Could you check a few things on this drawing? It's one solid part, dimensions in mm from its lowest x, y, z. A direction names the side the tool comes from. Give positions to 0.01 mm unless a question says otherwise; leave off trailing zeros. Order: outer loops, then holes, each group sorted by start corner. A loop starts at its lowest first (then second) coordinate and runs counter-clockwise, first axis right, second up.
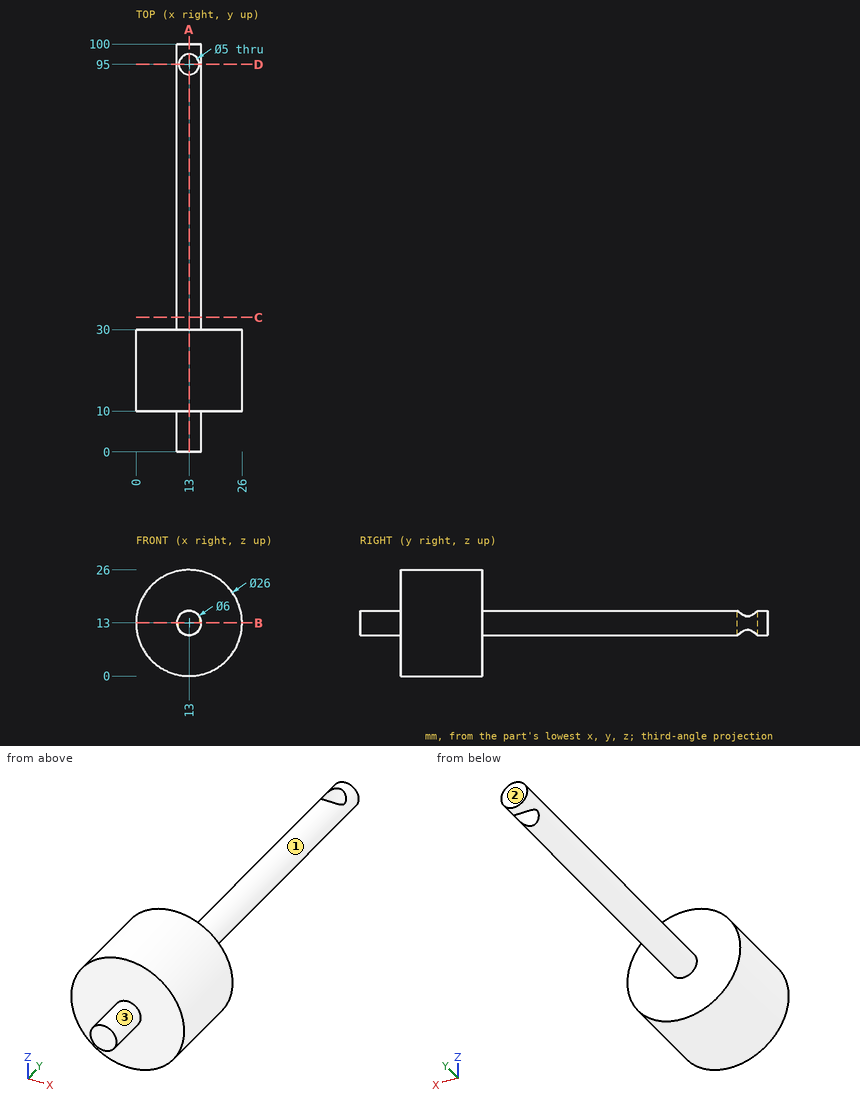
Q1. If we section it at B-B on z = 13: List the corners of the cut face in (x, y) for me.
Filled sheet:
outline: (0, 10) - (10, 10) - (10, 0) - (16, 0) - (16, 10) - (26, 10) - (26, 30) - (16, 30) - (16, 100) - (10, 100) - (10, 30) - (0, 30) - close; hole circle Ø5 at (13, 95)
Q2. I need wall thicknesses on L1, parallel to Y at x = 9.5, z = 6.75; L2, parallel to X at y = 95, z = 13.25; L3, parallel to Y at x = 13, z = 14. Which ranges of each line are inside material? Lowest first, please.
Filled sheet:
L1: y = 10 to 30
L2: x = 10.01 to 10.5, 15.5 to 15.99
L3: y = 0 to 92.5, 97.5 to 100
Q3. I'm going to push flat-ended pins straight in: P1, Ø12, axis at x = 19, y = 74, coming from the +Z side; P2, Ø8, axis at x = 6.5, y = 58, coming from the -Z side; P3, Ø12, axis at x = 5, z = 12.5, coming from the +Y side; P4, Ø5, axis at x = 20, z = 9, coming from the +Y side. Where does each tip first touch, or does it pass through?
Filled sheet:
P1: stops at z = 16
P2: stops at z = 11.34
P3: stops at y = 100
P4: stops at y = 30
Q4. If we section it at C-C on y = 33: List the corners of the cut face in (x, z) for me, plus the area to 3 significant figures.
Filled sheet:
outline: circle Ø6 at (13, 13)
area: 28.3 mm2
Q5. If we section it at D-D on y = 95: List the corners of the cut face in (x, z) for me, plus the area to 3 significant figures.
Filled sheet:
outline: (10.5, 11.34) - (10.5, 14.66) arc R3 ccw to start; (15.5, 11.34) arc R3 ccw to (15.5, 14.66) - close
area: 2.25 mm2
Q6. If we section it at A-A on x = 13: List the corners of the cut face in (y, z) for me, plus the area to 3 significant figures.
Filled sheet:
outline: (0, 10) - (10, 10) - (10, 0) - (30, 0) - (30, 10) - (92.5, 10) - (92.5, 16) - (30, 16) - (30, 26) - (10, 26) - (10, 16) - (0, 16) - close; (97.5, 10) - (100, 10) - (100, 16) - (97.5, 16) - close
area: 970 mm2
Q7. For the marked faces 1, 2 and 3, which set-ups out of +Z, -Z, +X, -X, +Y, -Y let a thin tool reach every point of the face, with its end or its side?
Filled sheet:
face 1: +Y
face 2: +Z, -Z, +X, -X, +Y
face 3: -Y
